from build123d import *

# Parameters (mm, degrees)
SKETCH_1_W          = 50
SKETCH_1_H          = 24
EXTRUDE_1_DEPTH     = 5
SKETCH_2_W          = 50
SKETCH_2_H          = 5
EXTRUDE_2_DEPTH     = 20
SKETCH_3_W          = 4
SKETCH_3_H          = 19
EXTRUDE_3_DEPTH     = 20
CUT_EXTRUDE_1_DEPTH = 50.497474683
SKETCH_6_R          = 1.1
CUT_EXTRUDE_2_DEPTH = 35.190641995
SKETCH_7_R          = 5
CUT_EXTRUDE_3_DEPTH = 43.731721238
SKETCH_8_R          = 1.6
CUT_EXTRUDE_4_DEPTH = 35.190641995
FILLET_1_R          = 8
CHAMFER_1_SIZE      = 1


with BuildPart() as part:
    # 草图1 → 凸台-拉伸1 (new body)
    with BuildSketch(Plane(origin=(0, 0, 0), x_dir=(1, 0, 0), z_dir=(0, 1, 0))):
        Rectangle(SKETCH_1_W, SKETCH_1_H)
    extrude(amount=EXTRUDE_1_DEPTH)

    # 草图2 → 凸台-拉伸2 (add)
    with BuildSketch(Plane(origin=(0, 5, 0), x_dir=(1, 0, 0), z_dir=(0, 1, 0))):
        with Locations((0, 9.5)):
            Rectangle(SKETCH_2_W, SKETCH_2_H)
    extrude(amount=EXTRUDE_2_DEPTH)

    # 草图3 → 凸台-拉伸3 (add)
    with BuildSketch(Plane(origin=(0, 5, 0), x_dir=(1, 0, 0), z_dir=(0, 1, 0))):
        with Locations((14, -2.5)):
            Rectangle(SKETCH_3_W, SKETCH_3_H)
        with Locations((-14, -2.5)):
            Rectangle(SKETCH_3_W, SKETCH_3_H)
    extrude(amount=EXTRUDE_3_DEPTH)

    # 草图4 → 切除-拉伸1 (cut, through all)
    with BuildSketch(Plane.ZY.offset(16)):
        Polygon((-7, 25), (12, 5), (12, 25), align=None)
    extrude(amount=-CUT_EXTRUDE_1_DEPTH, mode=Mode.SUBTRACT)

    # 草图6 → 切除-拉伸2 (cut, through all)
    with BuildSketch(Plane(origin=(0, 5, 0), x_dir=(1, 0, 0), z_dir=(0, 1, 0))):
        with Locations(Location((6, 4.25, 0), (0, 0, 270))):
            Circle(SKETCH_6_R)
        with Locations(Location((6, -3.75, 0), (0, 0, 270))):
            Circle(SKETCH_6_R)
        with Locations(Location((-6, 4.25, 0), (0, 0, 90))):
            Circle(SKETCH_6_R)
        with Locations(Location((-6, -3.75, 0), (0, 0, 90))):
            Circle(SKETCH_6_R)
    extrude(amount=-CUT_EXTRUDE_2_DEPTH, mode=Mode.SUBTRACT)

    # 草图7 → 切除-拉伸3 (cut, through all)
    with BuildSketch(Plane(origin=(0, 0, -12), x_dir=(-1, 0, 0), z_dir=(0, 0, -1))):
        with Locations((0, 15)):
            Circle(SKETCH_7_R)
    extrude(amount=-CUT_EXTRUDE_3_DEPTH, mode=Mode.SUBTRACT)

    # 草图8 → 切除-拉伸4 (cut, through all)
    with BuildSketch(Plane(origin=(0, 5, 0), x_dir=(1, 0, 0), z_dir=(0, 1, 0))):
        with Locations(Location((20, 1, 0), (0, 0, 270))):
            Circle(SKETCH_8_R)
        with Locations(Location((-20, 1, 0), (0, 0, 90))):
            Circle(SKETCH_8_R)
    extrude(amount=-CUT_EXTRUDE_4_DEPTH, mode=Mode.SUBTRACT)

    # 圆角1
    fillet_1_edges = [part.edges().sort_by_distance(p)[0] for p in [
        (-25, 25, -9.5),
        (25, 25, -9.5),
        (25, 2.5, 12),
        (-25, 2.5, 12),
    ]]
    fillet(fillet_1_edges, radius=FILLET_1_R)

    # 倒角1
    chamfer_1_edges = [part.edges().sort_by_distance(p)[0] for p in [
        (6, 5, 2.65),
        (-6, 5, -3.15),
        (-6, 5, 4.85),
        (6, 5, -5.35),
    ]]
    chamfer(chamfer_1_edges, length=CHAMFER_1_SIZE)


solid = part.part
Can you work these out from the model? Positions are in its coordinate system, mm. A direction names the side the tool comes from. Coordinates: 2 decimals unless noted, no trailing zeros. Loops run counter-clockwise (first coordinate to the right, second up) from the corner with the lowest first, then second, coordinate; pieces in that order, holes last. Notation, with made-up numbers: M 4,87 L 19,87 A5 ccw 19,96 Z; hole C -17.5,58.5 d4. An arc over 180 degrees is marked long. Answer as CSV lines item,"result". Start each with the question number.
1. If I drill on probe 1 along X at (y, z) = (2, 3.75); probe 2 along Z at (x, y) = (-6, 2.2); probe 3 along X at (y, z) = (21.25, -6), over which ranges is the centre line in solid material (lowest first)? Write a range as [from, to].
2. For pin 1 Ø6 at (y, z) = (17, 1) entering from +X; pin 2 Ø2.5 at (x, z) = (-6, -4.25) entering from +Y; pin 3 Ø2.5 at (x, z) = (22.5, 2) entering from +Y, each with a flat end and sliding along its axis, tell me the tip position at first contact or that it passes through.
3. Suppose I cut it at B-B, the plane x = 0. List the corners of the cut face in (y, z) for me, plus the area to 3 significant figures.
4. For faces 4 (the face through (-21, 15, -7)), 5 (the face through (16, 10, -2)), 6 (the face through (-3, 10, -7)), which set-ups out of +Z, -Z, +X, -X, +Y, -Y let a thin tool reach every point of the face, with its end or its side?
5. Suppose I cut it at D-D, the plane z = -1. List the corners of the cut face in (x, y) for me.
6. Thinking about a two-plate mould opening in X: for faces 1 (the face through (-6.33, 2.03, 2.7)), 2 (the face through (0, 25, -10)), 3 (the face through (-16, 10, -2)), which applies, +X half, -X half, draft (parallel to the pull), parting line (faces both ways), or undercut?
7. Suppose I cut it at C-C, the plane x = 6. List the corners of the cut face in (y, z) for me.
8. Suppose I cut it at A-A, the plane y = 15. List the corners of the cut face in (x, z) for me.
Output:
1,probe 1,"x = [-25, -7.1], [-4.9, 4.9], [7.1, 25]"
1,probe 2,"z = [-12, -5.35], [-3.15, 2.65], [4.85, 12]"
1,probe 3,"x = [-16, -12], [12, 16]"
2,pin 1,"stops at x = 16"
2,pin 2,"stops at y = 4.15"
2,pin 3,"stops at y = 5"
3,outline,"M 0,-12 L 10,-12 L 10,-7 L 5,-7 L 5,12 L 0,12 Z; M 20,-12 L 25,-12 L 25,-7 L 20,-7 Z"
3,area,"170 mm^2"
4,face 4,"+Z, -X, +Y"
4,face 5,"+Z, +X, +Y"
4,face 6,"+Z, +Y"
5,outline,"M -25,0 L -21.6,0 L -21.6,5 L -25,5 Z; M -18.4,0 L 18.4,0 L 18.4,5 L 16,5 L 16,18.68 L 12,18.68 L 12,5 L -12,5 L -12,18.68 L -16,18.68 L -16,5 L -18.4,5 Z; M 21.6,0 L 25,0 L 25,5 L 21.6,5 Z"
6,face 1,"undercut"
6,face 2,"draft"
6,face 3,"-X half"
7,outline,"M 0,-12 L 25,-12 L 25,-7 L 5,-7 L 5,-6.35 L 4,-5.35 L 0,-5.35 Z; M 0,-3.15 L 4,-3.15 L 5,-2.15 L 5,1.65 L 4,2.65 L 0,2.65 Z; M 0,4.85 L 4,4.85 L 5,5.85 L 5,12 L 0,12 Z"
8,outline,"M -25,-12 L -5,-12 L -5,-7 L -12,-7 L -12,2.5 L -16,2.5 L -16,-7 L -25,-7 Z; M 5,-12 L 25,-12 L 25,-7 L 16,-7 L 16,2.5 L 12,2.5 L 12,-7 L 5,-7 Z"
